```python
from build123d import *

# Parameters (mm, degrees)
SKETCH_W        = 40
SKETCH_H        = 40
PAD_DEPTH       = 80
SKETCH001_R     = 6.5
POCKET_DEPTH    = 30
SKETCH002_R     = 4.25
POCKET001_DEPTH = 55


with BuildPart() as part:
    # Sketch → Pad (new body)
    with BuildSketch(Plane.XY):
        Rectangle(SKETCH_W, SKETCH_H)
    extrude(amount=-PAD_DEPTH)

    # Sketch001 (on Face5 of Pad) → Pocket (cut)
    with BuildSketch(Plane.XY):
        Circle(SKETCH001_R)
    extrude(amount=-POCKET_DEPTH, mode=Mode.SUBTRACT)

    # Sketch002 (on Face4 of Pocket) → Pocket001 (cut)
    with BuildSketch(Plane.XY):
        Circle(SKETCH002_R)
    extrude(amount=-POCKET001_DEPTH, mode=Mode.SUBTRACT)


solid = part.part
```
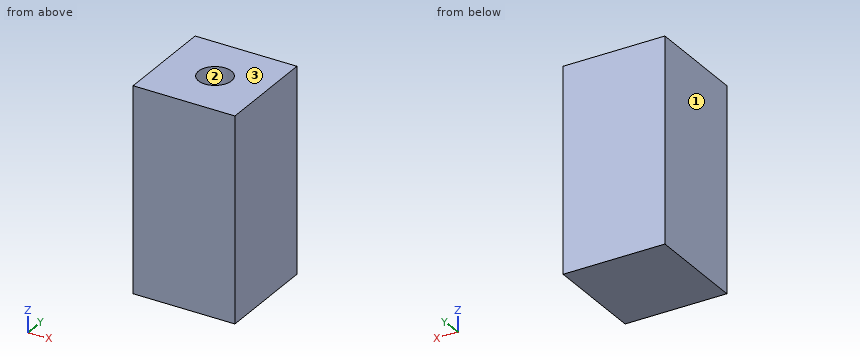
For this review, take the finished solid that the model builds, in its own axes (mm). Face numbers are marked on the shaded views. Coordinates: 2 decimals unless noted, no trailing zeros. Write each loop counter-clockwise with the first axis right and the second up, starting at its lowest first coordinate (ties: lowest second). Pieces come first, ordered by that corner, then holes.
(1) Add section D-D on z = -43. Give the boundary of the cut face in (x, y).
(2) Wall thickness on probe 1 along Y at (x, z) = (0, -14); probe 2 along Y at (x, z) = (0, -36); probe 3 along X at (y, z) = (-2, -38.5): over which ranges is each line inside the solid? List them lowest first.
(3) The part is to be moulded in two halves that separate along X. For the marked faces 1, 2 and 3, say which applies: +X half, -X half, draft (parallel to the pull), parting line (faces both ways), or undercut.
(4) For pin 1 Ø6 at (x, y) = (12, -2) entering from +Z; pin 2 Ø9.5 at (x, y) = (-0.5, -1.5) entering from +Z; pin 3 Ø8 at (x, y) = (0, 0) entering from +Z, all flat-tipped, find the tip position at first contact; note any pin that passes through.
(5) Add section A-A on z = -8. Give the boundary of the cut face in (x, y).
(6) Add section B-B on x = 0. Give the boundary of the cut face in (y, z).
Answer sheet:
1. outline: (-20, -20) - (20, -20) - (20, 20) - (-20, 20) - close; hole circle Ø8.5 at (0, 0)
2. probe 1: y = -20 to -6.5, 6.5 to 20
2. probe 2: y = -20 to -4.25, 4.25 to 20
2. probe 3: x = -20 to -3.75, 3.75 to 20
3. face 1: -X half
3. face 2: undercut
3. face 3: draft
4. pin 1: stops at z = 0
4. pin 2: stops at z = -30
4. pin 3: stops at z = -55
5. outline: (-20, -20) - (20, -20) - (20, 20) - (-20, 20) - close; hole circle Ø13 at (0, 0)
6. outline: (-20, -80) - (20, -80) - (20, 0) - (6.5, 0) - (6.5, -30) - (4.25, -30) - (4.25, -55) - (-4.25, -55) - (-4.25, -30) - (-6.5, -30) - (-6.5, 0) - (-20, 0) - close
